Could you check a few things on this model? Use its own coordinates, in mm. A direction names the side the tool comes from. Coordinates: 2 decimals unless noted, no trailing zeros. Loops run counter-clockwise (first coordinate to the right, second up) from the corner with the lowest first, then second, coordinate; pieces in that order, holes last.
Autodesk Inventor part; units mm, degrees
ref_plane "YZ Plane" through (0, 0, 0) normal (1, 0, 0) x (0, 1, 0)
ref_plane "XZ Plane" through (0, 0, 0) normal (0, 1, 0) x (-1, 0, 0)
ref_plane "XY Plane" through (0, 0, 0) normal (0, 0, 1) x (1, 0, 0)
sketch "Sketch1" plane through (0, 0, 0) normal (0, 1, 0) x (-1, 0, 0)
  line L0 (53.3, 0) -> (0, 0)
  line L1 (0, 0) -> (0, -65)
  line L2 (0, -65) -> (2, -65)
  line L3 (2, -65) -> (5, -68.6)
  line L4 (5, -68.6) -> (37, -68.6)
  line L5 (37, -68.6) -> (40, -65)
  line L6 (40, -65) -> (52.46, -65)
  line L7 (52.46, -65) -> (53.3, -64.3)
  line L8 (53.3, -64.3) -> (53.3, 0)
  line L9 (63.96, 0) -> (-10.66, 0)
  line L10 (0, -82.32) -> (0, 13.72)
  circle A0 centre (50.3, -15.1) radius 1.6
  circle A1 centre (2.5, -14) radius 1.6
  circle A2 centre (35.1, -65.9) radius 1.6
  circle A3 centre (7.2, -65.9) radius 1.6
  dimension "d2" = 53.3
  dimension "d5" = 51.9
  dimension "d6" = 1.1
  dimension "d8" = 27.9
  dimension "d9" = 15.2
  dimension "d10" = 68.6
  dimension "d11" = 3.2
  dimension "d12" = 50.8
  dimension "d13" = 4.7
  dimension "d15" = 2.5
  dimension "d17" = 14
  dimension "d18" = 37
  dimension "d19" = 40
  dimension "d20" = 2
  dimension "d21" = 5
  dimension "d22" = 65
extrude "board" add sketch "Sketch1" along normal blind 1.6
sketch "Sketch2" plane through (0, 1.6, 0) normal (0, 1, 0) x (1, 0, 0)
  line L0 (-43.7, -6.2) -> (-31.7, -6.2)
  line L1 (-31.7, -6.2) -> (-31.7, 7.8481)
  line L2 (-31.7, 7.8481) -> (-43.7, 7.8481)
  line L3 (-43.7, 7.8481) -> (-43.7, -6.2)
  line L4 (-12.2, -1.8) -> (-3.3, -1.8)
  line L5 (-3.3, -1.8) -> (-3.3, 12.0502)
  line L6 (-3.3, 12.0502) -> (-12.2, 12.0502)
  line L7 (-12.2, 12.0502) -> (-12.2, -1.8)
  line L8 (-50.0547, 22.1848) -> (-47.7065, 22.1848)
  line L9 (-47.7065, 22.1848) -> (-47.7065, 42.392)
  line L10 (-47.7065, 42.392) -> (-50.0547, 42.392)
  line L11 (-50.0547, 42.392) -> (-50.0547, 22.1848)
  line L12 (-50.0547, 43.9369) -> (-47.7065, 43.9369)
  line L13 (-47.7065, 43.9369) -> (-47.7065, 62.4757)
  line L14 (-47.7065, 62.4757) -> (-50.0547, 62.4757)
  line L15 (-50.0547, 62.4757) -> (-50.0547, 43.9369)
  line L16 (-3.9549, 32.1957) -> (-1.6067, 32.1957)
  line L17 (-1.6067, 32.1957) -> (-1.6067, 48.2627)
  line L18 (-1.6067, 48.2627) -> (-3.9549, 48.2627)
  line L19 (-3.9549, 48.2627) -> (-3.9549, 32.1957)
  line L20 (-3.9549, 49.2514) -> (-1.6067, 49.2514)
  line L21 (-1.6067, 49.2514) -> (-1.6067, 62.2285)
  line L22 (-1.6067, 62.2285) -> (-3.9549, 62.2285)
  line L23 (-3.9549, 62.2285) -> (-3.9549, 49.2514)
  line L24 (-53.3, 64.3) -> (-53.3, 0)
  line L25 (0, 0) -> (0, 65)
  line L26 (-53.3, 0) -> (0, 0)
  line L27 (-20.8879, 23.0716) -> (-10.5062, 23.0716)
  line L28 (-10.5062, 23.0716) -> (-10.5062, 62.2285)
  line L29 (-10.5062, 62.2285) -> (-20.8879, 62.2285)
  line L30 (-20.8879, 62.2285) -> (-20.8879, 23.0716)
  dimension "d25" = 9.6
  dimension "d26" = 12
  dimension "d27" = 3.3
  dimension "d28" = 8.9
  dimension "d29" = 1.8
  dimension "d30" = 6.2
extrude "Extrusion2" add sketch "Sketch2" along normal blind 10.9 contours L3 L26 L1 L0 | L7 L6 L5 L26 | L26 L5 L4 L7 | L3 L2 L1 L26
extrude "Extrusion3" add sketch "Sketch2" along normal blind 5 contours L30 L29 L28 L27
extrude "Extrusion4" add sketch "Sketch2" along normal blind 9 contours L11 L10 L9 L8 | L15 L14 L13 L12 | L19 L18 L17 L16 | L23 L22 L21 L20
properties part number "arduino_uno"
1) Imagine slicing it at D-D on x = -42. List the corners of the cut face in (y, z) for me.
2) Imagine slicing it at B-B on x = -7.2. List the corners of the cut face in (y, z) for me, plus the area to 3 significant figures.
3) Will these pins go through, and if not, where does the flat tip stop? pin 1 (4.5 mm diameter, centred on y = 8, z = -58.5, fed in from -X); pin 2 (0.7 mm diameter, centred on x = -3.5, z = -54.5, fed in from +Y); pin 3 (1.5 mm diameter, centred on x = -14, y = 3.5, fed in from +Z).
4) Imagine slicing it at A-A on y = 3.75. List the corners of the cut face in (x, z) for me, plus the area to 3 significant figures.
5) If I drill on L1, parallel to X at y = 5.25, z = -38; L2, parallel to Z at x = -7.2, y = 0.75; L3, parallel to Z at x = -50.3, y = 1.3, over which ranges is the centre line in solid material (lowest first)?
6) Imagine slicing it at C-C on z = -26.5. List the corners of the cut face in (x, y) for me, plus the area to 3 significant figures.
7) We'd pull the mould along Z, two halves only. Please class faces 6 (the flat face through (-16, 4, -62.228)), 7 (the flat face through (-31.7, 7, -1)), 8 (the flat face through (-3, 6, -48.263)): released by +Z, released by -Z, zero draft, split by the parting line, or undercut.
8) For faces 1 (the flat face through (-8, 7, -12.05)), 2 (the flat face through (-20.888, 4, -43)), 3 (the flat face through (-3.955, 6, -56)), 4 (the flat face through (-46, 1, -65)), 5 (the flat face through (-3, 10.6, -56)), which set-ups out of +Z, -Z, +X, -X, +Y, -Y let a thin tool reach every point of the face, with its end or its side?
Solved:
1. outline: (0, -65) - (1.6, -65) - (1.6, -7.85) - (12.5, -7.85) - (12.5, 6.2) - (1.6, 6.2) - (1.6, 0) - (0, 0) - close
2. outline: (0, -68.6) - (1.6, -68.6) - (1.6, -67.5) - (0, -67.5) - close; (0, -64.3) - (1.6, -64.3) - (1.6, -12.05) - (12.5, -12.05) - (12.5, 1.8) - (1.6, 1.8) - (1.6, 0) - (0, 0) - close
2. area: 256 mm2
3. pin 1: stops at x = -50.05
3. pin 2: stops at y = 10.6
3. pin 3: stops at z = -23.07
4. outline: (-50.05, -62.48) - (-47.71, -62.48) - (-47.71, -43.94) - (-50.05, -43.94) - close; (-50.05, -42.39) - (-47.71, -42.39) - (-47.71, -22.18) - (-50.05, -22.18) - close; (-43.7, -7.85) - (-31.7, -7.85) - (-31.7, 6.2) - (-43.7, 6.2) - close; (-20.89, -62.23) - (-10.51, -62.23) - (-10.51, -23.07) - (-20.89, -23.07) - close; (-12.2, -12.05) - (-3.3, -12.05) - (-3.3, 1.8) - (-12.2, 1.8) - close; (-3.95, -62.23) - (-1.61, -62.23) - (-1.61, -49.25) - (-3.95, -49.25) - close; (-3.95, -48.26) - (-1.61, -48.26) - (-1.61, -32.2) - (-3.95, -32.2) - close
4. area: 858 mm2
5. L1: x = -50.05 to -47.71, -20.89 to -10.51, -3.95 to -1.61
5. L2: z = -68.6 to -67.5, -64.3 to 0
5. L3: z = -65 to -16.7, -13.5 to 0
6. outline: (-53.3, 0) - (0, 0) - (0, 1.6) - (-10.51, 1.6) - (-10.51, 6.6) - (-20.89, 6.6) - (-20.89, 1.6) - (-47.71, 1.6) - (-47.71, 10.6) - (-50.05, 10.6) - (-50.05, 1.6) - (-53.3, 1.6) - close
6. area: 158 mm2
7. face 6: released by -Z
7. face 7: zero draft
7. face 8: undercut
8. face 1: +X, -X, +Y
8. face 2: +Z, -Z, +Y
8. face 3: -Z, +Y
8. face 4: -Z, -X, +Y, -Y
8. face 5: -Z, +X, -X, +Y
